The model under review builds one solid part; all positions refer to its coordinate system, in mm. A direction names the side the tool comes from. Round coordinates to 2 decimals unless told otherwise and drop trailing zeros. Write each loop counter-clockwise with the first axis right and the second up, starting at its lowest first coordinate (ties: lowest second). Pieces come first, ordered by that corner, then holes. Notation, with made-up numbers: M 44.5,86.5 L 90.5,86.5 A26 cw 90.5,109.5 Z; hole C 23.5,41.5 d5. An arc over 180 degrees is marked long. One line per item, written item: value. Start each with the question number.
1) Take a section at B-B, the plane x = 30. Write out the cut boundary in (y, z), and give its area (3 significant figures).
2) Take a section at A-A, the plane y = 40. Write out the cut boundary in (x, z), and give its area (3 significant figures).
3) Tool access review of faces 3 (the face through (-3.11, 34.01, 1.18)), 4 (the face through (-40, 1, 12)), 5 (the face through (20, 45, 30)), 6 (the face through (30, -45, 45)), 7 (the face through (-2.17, -49.76, 8.79)): name each direction out of +Z, -Z, +X, -X, +Y, -Y from which nothing blocks a thin tool from reaching the whole face with its end or side.
4) Take a section at D-D, the plane z = 6.5. Write out the cut boundary in (x, y).
5) Take a section at C-C, the plane x = 0. Write out the cut boundary in (y, z), and give its area (3 significant figures).
6) Wall thickness on probe 1 along Y at (x, z) = (0, 1.9); probe 2 along Y at (x, z) = (-30, 10); probe 3 along Y at (x, z) = (-24, 18): over which ranges is each line inside the solid? List them lowest first.
7) Mouldability with a two-part tool opening along Y and no side actions: class faces 1 (the face through (-20, 45, 30)), 2 (the face through (-3.63, -34.31, 1.18)) as +Y half, -Y half, draft (parallel to the pull), parting line (faces both ways), or undercut.
8) For P1, Ø10, axis at x = 2, y = 42, coming from the +Z side; P2, Ø1, axis at x = -24, y = -8.5, coming from the +Z side; P3, Ø5.5, axis at x = 27.5, y = 0.5, coming from the +Z side, all flat-tipped, find the tip position at first contact; note any pin that passes through.
from build123d import *

# Parameters (mm, degrees)
SKETCH_1_W                    = 80
SKETCH_1_H                    = 110
EXTRUDE_1_DEPTH               = 15
HOLE_WIZARD_M12_1_D           = 13.5
HOLE_WIZARD_M12_1_CBORE_D     = 20
HOLE_WIZARD_M12_1_CBORE_DEPTH = 12.6
EXTRUDE_2_DEPTH               = 20
SKETCH_5_R                    = 5
CUT_EXTRUDE_1_DEPTH           = 10
HOLE_WIZARD_M6_1_D            = 6.6
HOLE_WIZARD_M6_1_CBORE_D      = 11
HOLE_WIZARD_M6_1_CBORE_DEPTH  = 6.4


with BuildPart() as part:
    # 草图1 → 凸台-拉伸1 (new body)
    with BuildSketch(Plane.XY):
        Rectangle(SKETCH_1_W, SKETCH_1_H)
    extrude(amount=EXTRUDE_1_DEPTH)

    # M12 六角凹头螺钉的柱形沉头孔1 (through all)
    with Locations(Plane.XY.offset(15)):
        with Locations((0, 40), (0, -40)):
            CounterBoreHole(HOLE_WIZARD_M12_1_D / 2, HOLE_WIZARD_M12_1_CBORE_D / 2, HOLE_WIZARD_M12_1_CBORE_DEPTH)

    # 草图4 → 凸台-拉伸2 (add)
    with BuildSketch(Plane.XZ.offset(55)):
        with BuildLine():
            Line((-40, 15), (-40, 45))
            ThreePointArc((-40, 45), (-30, 55), (-20, 45))
            Line((-20, 45), (-20, 15))
            Line((-20, 15), (-40, 15))
        make_face()
        with BuildLine():
            Line((40, 15), (40, 45))
            ThreePointArc((40, 45), (30, 55), (20, 45))
            Line((20, 45), (20, 15))
            Line((20, 15), (40, 15))
        make_face()
    extrude_2 = extrude(amount=-EXTRUDE_2_DEPTH)

    # 镜向1: 凸台-拉伸2 across plane
    add(extrude_2.mirror(Plane(origin=(0, 0, 0), x_dir=(0, 0, 1), z_dir=(0, -1, 0))))

    # 草图5 → 切除-拉伸1 (cut)
    with BuildSketch(Plane(origin=(0, -35, 0), x_dir=(1, 0, 0), z_dir=(0, 1, 0))):
        with Locations(Location((30, -45, 0), (0, 0, 270))):
            Circle(SKETCH_5_R)
        with Locations(Location((-30, -45, 0), (0, 0, 270))):
            Circle(SKETCH_5_R)
    cut_extrude_1 = extrude(amount=-CUT_EXTRUDE_1_DEPTH, mode=Mode.SUBTRACT)

    # 镜向2: 切除-拉伸1 across plane
    add(cut_extrude_1.mirror(Plane(origin=(0, 0, 0), x_dir=(0, 0, 1), z_dir=(0, -1, 0))), mode=Mode.SUBTRACT)

    # M6 六角凹头螺钉的柱形沉头孔1 (through all)
    with Locations(Plane.XY.offset(15)):
        with Locations((-30, 0), (30, 0)):
            CounterBoreHole(HOLE_WIZARD_M6_1_D / 2, HOLE_WIZARD_M6_1_CBORE_D / 2, HOLE_WIZARD_M6_1_CBORE_DEPTH)


solid = part.part
Checked values:
1. outline: M -55,0 L -3.3,0 L -3.3,8.6 L -5.5,8.6 L -5.5,15 L -35,15 L -35,40 L -45,40 L -45,50 L -35,50 L -35,55 L -55,55 Z; M 3.3,0 L 55,0 L 55,55 L 35,55 L 35,50 L 45,50 L 45,40 L 35,40 L 35,15 L 5.5,15 L 5.5,8.6 L 3.3,8.6 Z
1. area: 2,920 mm2
2. outline: M -40,0 L -6.75,0 L -6.75,2.4 L -10,2.4 L -10,15 L -20,15 L -20,45 A10 ccw -40,45 Z; M 6.75,0 L 40,0 L 40,45 A10 ccw 20,45 L 20,15 L 10,15 L 10,2.4 L 6.75,2.4 Z; hole C -30,45 d10; hole C 30,45 d10
2. area: 2,270 mm2
3. face 3: +Z, -Z
3. face 4: +Z, -Z, -X, +Y, -Y
3. face 5: +Z, +Y, -Y
3. face 6: none
3. face 7: +Z
4. outline: M -40,-55 L 40,-55 L 40,55 L -40,55 Z; hole C -30,0 d6.6; hole C 0,-40 d20; hole C 0,40 d20; hole C 30,0 d6.6
5. outline: M -55,0 L -46.75,0 L -46.75,2.4 L -50,2.4 L -50,15 L -55,15 Z; M -33.25,0 L 33.25,0 L 33.25,2.4 L 30,2.4 L 30,15 L -30,15 L -30,2.4 L -33.25,2.4 Z; M 46.75,0 L 55,0 L 55,15 L 50,15 L 50,2.4 L 46.75,2.4 Z
5. area: 1,080 mm2
6. probe 1: y = -55 to -46.75, -33.25 to 33.25, 46.75 to 55
6. probe 2: y = -55 to -5.5, 5.5 to 55
6. probe 3: y = -55 to -35, 35 to 55
7. face 1: draft
7. face 2: undercut
8. P1: stops at z = 2.4
8. P2: stops at z = 15
8. P3: stops at z = 8.6
